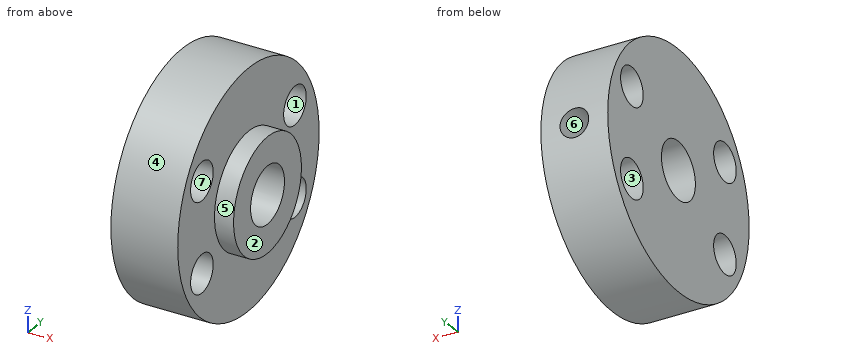
from build123d import *

# Parameters (mm, degrees)
ESQUISSE2_R             = 2
ENL_V_MAT_EXTRU_1_DEPTH = 8
ESQUISSE3_R             = 1.5
ENL_V_MAT_EXTRU_2_DEPTH = 30


with BuildPart() as part:
    # Esquisse1 → Révolution1 (revolve)
    with BuildSketch(Plane.XY):
        Polygon((0, 3), (0, 12.5), (7, 12.5), (7, 6), (9, 6), (9, 3), align=None)
    revolve(axis=Axis((0, 0, 0), (1, 0, 0)))

    # Esquisse2 → Enlèv. mat.-Extru.1 (cut, through all)
    with BuildSketch(Plane(origin=(7, 0, 0), x_dir=(0, 0, -1), z_dir=(1, 0, 0))):
        with Locations((-4.75, 8.227241336)):
            Circle(ESQUISSE2_R)
        with Locations((4.75, 8.227241336)):
            Circle(ESQUISSE2_R)
        with Locations((-4.75, -8.227241336)):
            Circle(ESQUISSE2_R)
        with Locations((4.75, -8.227241336)):
            Circle(ESQUISSE2_R)
    extrude(amount=-ENL_V_MAT_EXTRU_1_DEPTH, mode=Mode.SUBTRACT)

    # Esquisse3 → Enlèv. mat.-Extru.2 (cut)
    with BuildSketch(Plane(origin=(0, 0, 0), x_dir=(1, 0, 0), z_dir=(0, 1, 0))):
        with Locations((3.5, 0)):
            Circle(ESQUISSE3_R)
    extrude(amount=ENL_V_MAT_EXTRU_2_DEPTH, mode=Mode.SUBTRACT)


solid = part.part
Design review of the part built by this model. Coordinates are the model's own, in mm. Face numbers are marked on the shaded views. A direction names the side the tool comes from. Coordinates: 2 decimals unless noted, no trailing zeros. Write each loop counter-clockwise with the first axis right and the second up, starting at its lowest first coordinate (ties: lowest second). Pieces come first, ordered by that corner, then holes. Notation, with made-up numbers: (23.25, 60) - (29.25, 60) arc R22 ccw to (29.25, 80) - close; hole circle Ø4 at (80.25, -26). An arc over 180 degrees is marked (long way). One line per item, written item: value.
1) Add section C-C (y = -7). State the section outline as (x, z) points.
Answer sheet:
outline: (0, -10.36) - (7, -10.36) - (7, -6.33) - (0, -6.33) - close; (0, -3.17) - (7, -3.17) - (7, 3.17) - (0, 3.17) - close; (0, 6.33) - (7, 6.33) - (7, 10.36) - (0, 10.36) - close
2) Mouldability with a two-part tool opening along Z and no side actions: class the marked faces 1, 2, 3 and 4 as +Z half, -Z half, draft (parallel to the pull), parting line (faces both ways), or undercut.
Answer sheet:
face 1: undercut
face 2: draft
face 3: undercut
face 4: parting line
3) Insertion check: pin 1 (9.5 mm diameter, centred on y = 0, z = 0, fed in from +X); pin 2 (2.5 mm diameter, centred on y = 8.23, z = -4.75, fed in from +X); pin 3 (1.8 mm diameter, centred on x = 3.5, z = 0, fed in from +Y); pin 4 (5 mm diameter, centred on y = -8.23, z = 4.75, fed in from +X). Each pin has a flat end and moves straight along its axis. Give the tip position at first contact, or say it passes through.
Answer sheet:
pin 1: stops at x = 9
pin 2: passes through
pin 3: stops at y = -2.86
pin 4: stops at x = 7
4) Add section B-B (y = 0). State the section outline as (x, z) points.
Answer sheet:
outline: (0, -12.5) - (7, -12.5) - (7, -6) - (9, -6) - (9, -3) - (0, -3) - close; (0, 3) - (9, 3) - (9, 6) - (7, 6) - (7, 12.5) - (0, 12.5) - close
5) For the marked faces 5, 6 and 7, list the 3-axis set-ups (+Z, -Z, +X, -X, +Y, -Y) from which the entire face can be reached by the end or side of a thin tool; tool diameter is ignored.
Answer sheet:
face 5: +X
face 6: +Y
face 7: +X, -X
6) Add section A-A (z = 0). State the section outline as (x, y) points.
Answer sheet:
outline: (0, -12.5) - (7, -12.5) - (7, -6) - (9, -6) - (9, -3) - (0, -3) - close; (0, 3) - (2, 3) - (2, 12.5) - (0, 12.5) - close; (5, 3) - (9, 3) - (9, 6) - (7, 6) - (7, 12.5) - (5, 12.5) - close
7) Add section D-D (x = 6.5). State the section outline as (y, z) points.
Answer sheet:
outline: circle Ø25 at (0, 0); hole circle Ø4 at (-8.23, -4.75); hole circle Ø4 at (-8.23, 4.75); hole circle Ø6 at (0, 0); hole circle Ø4 at (8.23, -4.75); hole circle Ø4 at (8.23, 4.75)
8) To check wall thickness, follow probe 1 along Z at (x, y) = (5.5, 0); probe 2 along Z at (x, y) = (3, 7.25) (3 decimals); probe 3 along Y at (x, z) = (5, -4.75). State the ranges of each line that lie inside material, in increasing order.
Answer sheet:
probe 1: z = -12.5 to -3, 3 to 12.5
probe 2: z = -10.183 to -6.495, -3.005 to -1.414, 1.414 to 3.005, 6.495 to 10.183
probe 3: y = -11.56 to -10.23, -6.23 to 6.23, 10.23 to 11.56
